from build123d import *

# Parameters (mm, degrees)
SKETCH1_W           = 7.2
SKETCH1_H           = 5.4
STEM_HOUSING_DEPTH  = 4.5
SKETCH3_W           = 7.2
SKETCH3_H           = 5.4
BOSS_EXTRUDE2_DEPTH = 1.6
FILLET2_R           = 1


with BuildPart() as part:
    # Sketch1 → stem housing (new body)
    with BuildSketch(Plane(origin=(0, 0, 0), x_dir=(1, 0, 0), z_dir=(0, 1, 0))):
        Rectangle(SKETCH1_W, SKETCH1_H)
        with BuildLine():
            Line((-0.675, 0.975), (-0.675, 2.1))
            Line((-0.675, 2.1), (0.675, 2.1))
            Line((0.675, 2.1), (0.675, 0.975))
            ThreePointArc((0.675, 0.975), (0.762867966, 0.762867966), (0.975, 0.675))
            Line((0.975, 0.675), (2.15, 0.675))
            Line((2.15, 0.675), (2.15, -0.675))
            Line((2.15, -0.675), (0.975, -0.675))
            ThreePointArc((0.975, -0.675), (0.762867966, -0.762867966), (0.675, -0.975))
            Line((0.675, -0.975), (0.675, -2.1))
            Line((0.675, -2.1), (-0.675, -2.1))
            Line((-0.675, -2.1), (-0.675, -0.975))
            ThreePointArc((-0.675, -0.975), (-0.762867966, -0.762867966), (-0.975, -0.675))
            Line((-0.975, -0.675), (-2.15, -0.675))
            Line((-2.15, -0.675), (-2.15, 0.675))
            Line((-2.15, 0.675), (-0.975, 0.675))
            ThreePointArc((-0.975, 0.675), (-0.762867966, 0.762867966), (-0.675, 0.975))
        make_face(mode=Mode.SUBTRACT)
    extrude(amount=STEM_HOUSING_DEPTH)

    # Sketch3 → Boss-Extrude2 (add)
    with BuildSketch(Plane(origin=(0, 4.5, 0), x_dir=(1, 0, 0), z_dir=(0, 1, 0))):
        Rectangle(SKETCH3_W, SKETCH3_H)
    extrude(amount=BOSS_EXTRUDE2_DEPTH)

    # Fillet2
    fillet2_edges = [part.edges().sort_by_distance(p)[0] for p in [
        (-3.6, 3.05, 2.7),
        (-3.6, 3.05, -2.7),
        (3.6, 3.05, -2.7),
        (3.6, 3.05, 2.7),
    ]]
    fillet(fillet2_edges, radius=FILLET2_R)

    # Cut-Sweep1: sweep along a path in Sketch6
    with BuildLine(Plane(origin=(0, 6.1, 0), x_dir=(1, 0, 0), z_dir=(0, 1, 0))) as cut_sweep1_path:
        Line((-2.6, -2.7), (2.6, -2.7))
        ThreePointArc((2.6, -2.7), (3.307106781, -2.407106781), (3.6, -1.7))
        Line((3.6, -1.7), (3.6, 1.7))
        ThreePointArc((3.6, 1.7), (3.307106781, 2.407106781), (2.6, 2.7))
        Line((2.6, 2.7), (-2.6, 2.7))
        ThreePointArc((-2.6, 2.7), (-3.307106781, 2.407106781), (-3.6, 1.7))
        Line((-3.6, 1.7), (-3.6, -1.7))
        ThreePointArc((-3.6, -1.7), (-3.307106781, -2.407106781), (-2.6, -2.7))
    # Sketch4 → Cut-Sweep1 (sweep, cut)
    with BuildSketch(Plane.XY):
        with BuildLine():
            Line((-2.861522369, 6.1), (-3.061522369, 5.9))
            ThreePointArc((-3.061522369, 5.9), (-3.460054223, 5.30355493), (-3.6, 4.6))
            Line((-3.6, 4.6), (-3.6, 6.1))
            Line((-3.6, 6.1), (-2.861522369, 6.1))
        make_face()
    sweep(path=cut_sweep1_path.line, mode=Mode.SUBTRACT)


solid = part.part
The model under review builds one solid part; all positions refer to its coordinate system, in mm. A direction names the side the tool comes from. Round coordinates to 2 decimals unless told otherwise and drop trailing zeros. Loops run counter-clockwise (first coordinate to the right, second up) from the corner with the lowest first, then second, coordinate; pieces in that order, holes last. Notation, with made-up numbers: M -5,-35 L 34,-35 A26 ccw 34,4 Z; hole C 1.25,84.25 d4. An arc over 180 degrees is marked long. Answer as a JSON object with one key per item and string values.
Item 1: We need section A-A, the plane x = -2.5. State the section outline as (y, z) points, and give its area (3 significant figures).
Check sheet entries:
{"outline": "M 0,-2.7 L 4.6,-2.7 A1.84 ccw 5.9,-2.16 L 6.1,-1.96 L 6.1,1.96 L 5.9,2.16 A1.84 ccw 4.6,2.7 L 0,2.7 Z", "area": "32.2 mm2"}
Item 2: Tool access review of faces 4 (the face through (-1.6, 2.2, 0.675)), 5 (the face through (3.315, 2.268, -2.399)): name each direction out of +Z, -Z, +X, -X, +Y, -Y from which nothing blocks a thin tool from reaching the whole face with its end or side.
Check sheet entries:
{"face 4": "-Y", "face 5": "-Z, +X, +Y, -Y"}
Item 3: The part is to be moulded in two halves that separate along Z. For faces 1 (the face through (3.456, 5.313, -0.024)), 2 (the face through (-0.675, 2.2, 1.5)), 3 (the face through (-3.315, 2.268, -2.399)), say which applies: +Z half, -Z half, draft (parallel to the pull), parting line (faces both ways), or undercut.
Check sheet entries:
{"face 1": "draft", "face 2": "undercut", "face 3": "-Z half"}
Item 4: We need section B-B, the plane z = -1.5. State the section outline as (x, y) points (3 decimals).
Check sheet entries:
{"outline": "M -3.6,0 L -0.675,0 L -0.675,4.5 L 0.675,4.5 L 0.675,0 L 3.6,0 L 3.6,4.6 A1.838 ccw 3.062,5.9 L 2.862,6.1 L -2.862,6.1 L -3.062,5.9 A1.838 ccw -3.6,4.6 Z"}
Item 5: For line 1 along Z through (x, y) = (-1.5, 3) (3 decimals); line 2 along Z through (x, y) = (0.5, 0.5); line 3 along X through (y, z) = (1, 0.3), list the stretches that pass through material, from the lowest coordinate up.
Check sheet entries:
{"line 1": "-2.7 to -0.675, 0.675 to 2.7", "line 2": "-2.7 to -2.1, 2.1 to 2.7", "line 3": "-3.6 to -2.15, 2.15 to 3.6"}
Item 6: We need section D-D, the plane x = -0.5. State the section outline as (y, z) points.
Check sheet entries:
{"outline": "M 0,-2.7 L 4.6,-2.7 A1.84 ccw 5.9,-2.16 L 6.1,-1.96 L 6.1,1.96 L 5.9,2.16 A1.84 ccw 4.6,2.7 L 0,2.7 L 0,2.1 L 4.5,2.1 L 4.5,-2.1 L 0,-2.1 Z"}
Item 7: We need section C-C, the plane y = 3.75. State the section outline as (x, z) points (3 decimals).
Check sheet entries:
{"outline": "M -3.6,-1.7 A1 ccw -2.6,-2.7 L 2.6,-2.7 A1 ccw 3.6,-1.7 L 3.6,1.7 A1 ccw 2.6,2.7 L -2.6,2.7 A1 ccw -3.6,1.7 Z; hole M -2.15,-0.675 L -0.975,-0.675 A0.3 cw -0.675,-0.975 L -0.675,-2.1 L 0.675,-2.1 L 0.675,-0.975 A0.3 cw 0.975,-0.675 L 2.15,-0.675 L 2.15,0.675 L 0.975,0.675 A0.3 cw 0.675,0.975 L 0.675,2.1 L -0.675,2.1 L -0.675,0.975 A0.3 cw -0.975,0.675 L -2.15,0.675 Z"}
